Source: CAD feature listing. Evaluate the final solid. Frame: model axes, mm. Face numbers are marked on the shaded views. A direction names the side the tool comes from. Coordinates: 2 decimals unless noted, no trailing zeros. Order: outer loops, then holes, each group sorted by start corner. A loop starts at its lowest first (then second) coordinate and runs counter-clockwise, first axis right, second up.
Item 1: Section D-D on z = -3.75. Return the cut outline in (x, y), then the cut area to 3 significant figures.
Item 2: Ray query, line 1 (Y direction, x = 4, z = 3.25); line 2 (Z direction, x = 4.75, y = 7); line 3 (Z direction, x = 1.25, y = 22.5). Return the intervals inside material, ascending.
Item 3: Section B-B on x = 0. Return the cut outline in (y, z).
Item 4: Section A-A on z = 0. Return the cut outline in (x, y), then the cut area to 3 significant figures.
Item 5: Contact query for flat-ended pins moving along their axis: P1, Ø1, axis at x = 0, y = 22, coming from the -Z side; P2, Ø2, axis at x = 3, z = 4.5, coming from the +Y side. Output: stop coordinate, or through.
Item 6: Section C-C on y = 20.25. Return the cut outline in (x, z).
Item 7: Reachability of the marked faces 1 and 2 from +Z, -Z, +X, -X, +Y, -Y: full face, straight path, thin tool, end or side. Return the list, or none.
from build123d import *

# Parameters (mm, degrees)
CROQUIS1_W              = 10
CROQUIS1_H              = 12
SALIENTE_EXTRUIR1_DEPTH = 18
SALIENTE_EXTRUIR2_DEPTH = 6
REDONDEO1_R             = 1


with BuildPart() as part:
    # Croquis1 → Saliente-Extruir1 (new body)
    with BuildSketch(Plane(origin=(0, 0, 0), x_dir=(1, 0, 0), z_dir=(0, 1, 0))):
        Rectangle(CROQUIS1_W, CROQUIS1_H)
    extrude(amount=SALIENTE_EXTRUIR1_DEPTH)

    # Croquis2 → Saliente-Extruir2 (add)
    with BuildSketch(Plane(origin=(0, 18, 0), x_dir=(1, 0, 0), z_dir=(0, 1, 0))):
        with BuildLine():
            Line((-1.732050808, 1), (1.732050808, 1))
            ThreePointArc((1.732050808, 1), (0, -2), (-1.732050808, 1))
        make_face()
    extrude(amount=SALIENTE_EXTRUIR2_DEPTH)

    # Redondeo1
    redondeo1_edges = [part.edges().sort_by_distance(p)[0] for p in [
        (5, 9, 6),
        (-5, 9, 6),
        (-5, 9, -6),
        (5, 9, -6),
    ]]
    fillet(redondeo1_edges, radius=REDONDEO1_R)


solid = part.part
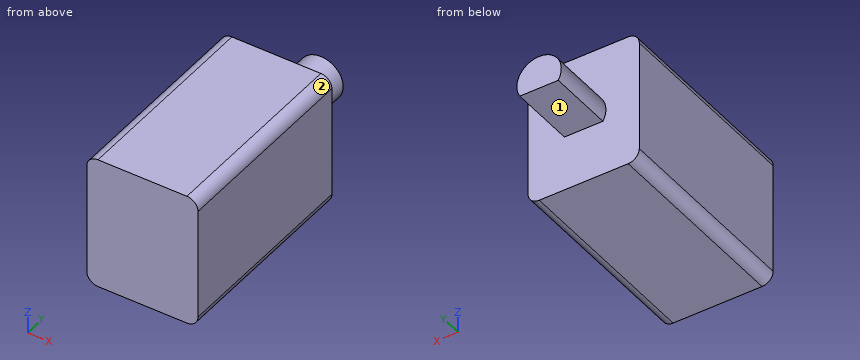
Answer list:
1. outline: (-5, 0) - (5, 0) - (5, 18) - (-5, 18) - close
1. area: 180 mm2
2. line 1: y = 0 to 18
2. line 2: z = -5.66 to 5.66
2. line 3: z = -1 to 1.56
3. outline: (0, -6) - (18, -6) - (18, -1) - (24, -1) - (24, 2) - (18, 2) - (18, 6) - (0, 6) - close
4. outline: (-5, 0) - (5, 0) - (5, 18) - (2, 18) - (2, 24) - (-2, 24) - (-2, 18) - (-5, 18) - close
4. area: 204 mm2
5. P1: stops at z = -1
5. P2: stops at y = 18
6. outline: (-1.73, -1) - (1.73, -1) arc R2 ccw (long way) to start
7. face 1: -Z, +X, -X, +Y
7. face 2: +Z, +X, +Y, -Y
